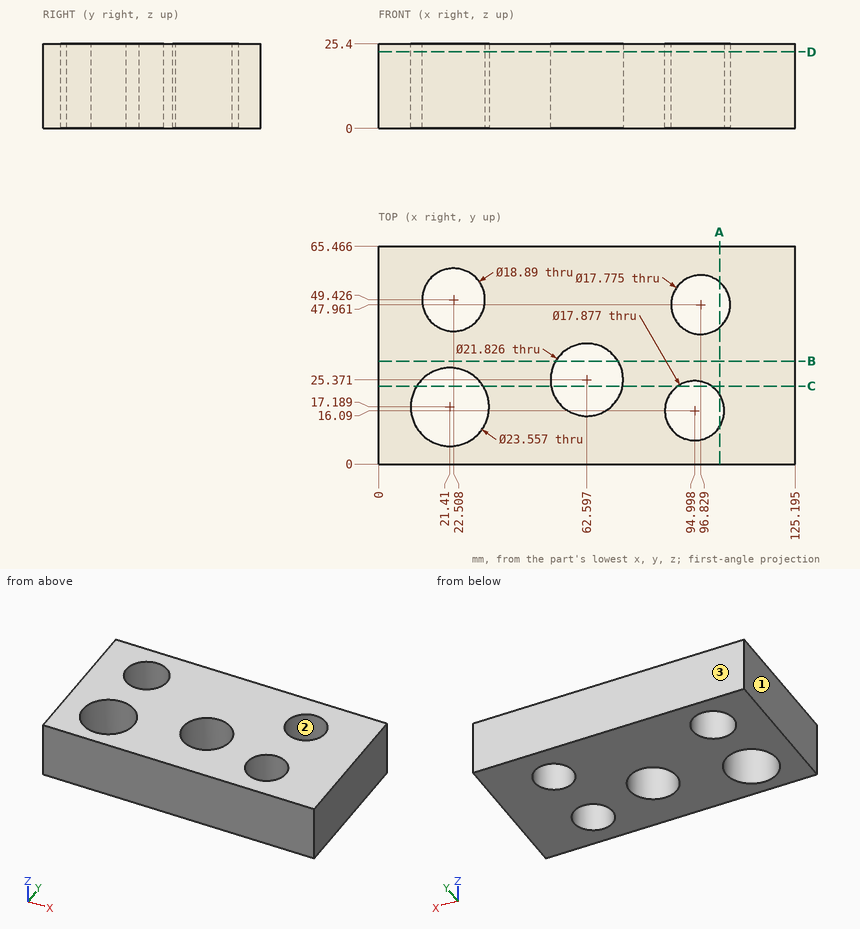
Geometry check sheet. Reference: drawing and pictorial views, mm from the part's lowest x, y, z. Give positions to 0.01 mm unless a question says otherwise; leave off trailing zeros. Order: outer loops, then holes, each group sorted by start corner. A loop starts at its lowest first (then second) coordinate and runs counter-clockwise, first axis right, second up. Notation, with made-up numbers: M -4,80.5 L 37,80.5 A27 ccw 37,110.5 Z; hole C -7,-32.5 d4. An arc over 180 degrees is marked long. Answer as a JSON object with one key per item and string values. Group by question number.
1) Cross-section at D-D (z = 23). Enter the section's corners in (x, y) (1 decimal).
2) Cross-section at C-C (y = 23.5). Enter the section's corners in (x, z) (1 decimal).
3) Scan lines: line 1 along X through (y, z) = (28, 12.25) (1 decimal); line 2 along X through (y, z) = (17.5, 18.5) (1 decimal); line 3 along X through (y, z) = (13, 22) (1 decimal). Record each from-to range of solid material in increasing order. Write a range as [from, to].
4) Mould release check, pull along Y, two halves, no side actions. Record for the marked faces 1, 2 and 3: released by +Y, released by -Y, zero draft, split by the parting line, or undercut.
5) Cross-section at A-A (x = 102.5). Give the number of separate pieces and of enclosed holes in the cut face, then the cut area to 3 significant figures.
6) Cross-section at B-B (y = 31). Enter the section's corners in (x, z) (1 decimal), then the cut area to 4 significant figures.
Result sheet:
{
 "1": {"outline": "M 0,0 L 125.2,0 L 125.2,65.5 L 0,65.5 Z; hole C 21.4,17.2 d23.6; hole C 22.5,49.4 d18.9; hole C 62.6,25.4 d21.8; hole C 95,16.1 d17.9; hole C 96.8,48 d17.8"},
 "2": {"outline": "M 0,0 L 11.5,0 L 11.5,25.4 L 0,25.4 Z; M 31.4,0 L 51.8,0 L 51.8,25.4 L 31.4,25.4 Z; M 73.3,0 L 90,0 L 90,25.4 L 73.3,25.4 Z; M 100,0 L 125.2,0 L 125.2,25.4 L 100,25.4 Z"},
 "3": {"line 1": "x = [0, 16.7], [26.1, 52], [73.2, 125.2]", "line 2": "x = [0, 9.6], [33.2, 55], [70.2, 86.2], [103.8, 125.2]", "line 3": "x = [0, 10.4], [32.4, 86.6], [103.4, 125.2]"},
 "4": {"face 1": "zero draft", "face 2": "undercut", "face 3": "released by +Y"},
 "5": {"separate pieces": "3", "enclosed holes": "0", "area": "1,070 mm2"},
 "6": {"outline": "M 0,0 L 53.2,0 L 53.2,25.4 L 0,25.4 Z; M 71.9,0 L 125.2,0 L 125.2,25.4 L 71.9,25.4 Z", "area": "2,705 mm2"}
}
